Geometry check sheet. Reference: drawing and pictorial views, mm from the part's lowest x, y, z. Give positions to 0.01 mm unless a question says otherwise; leave off trailing zeros. Write each loop counter-clockwise with the first axis right and the second up, starting at its lowest first coordinate (ties: lowest second). Pieces come first, ordered by that corner, then holes. Notation, with made-up numbers: M 76.5,58.5 L 104.5,58.5 A17 cw 104.5,63.5 Z; hole C 84,12 d5. An arc over 180 degrees is marked long. One line per item, written item: value. Start each with the question number.
1. Cross-section at B-B on x = 6.25. Record the cut outline in (y, z), then the cut area to 3 significant figures.
2. Cross-section at A-A on y = 1.7. Record the cut outline in (x, z), then the cut area to 3 significant figures.
3. Scan lines: line 1 (Z direction, x = 6, y = 3.2); line 2 (Z direction, x = 4.5, y = 1.1); line 3 (Y direction, x = 5, z = 7). Record each from-to range of solid material in increasing order.
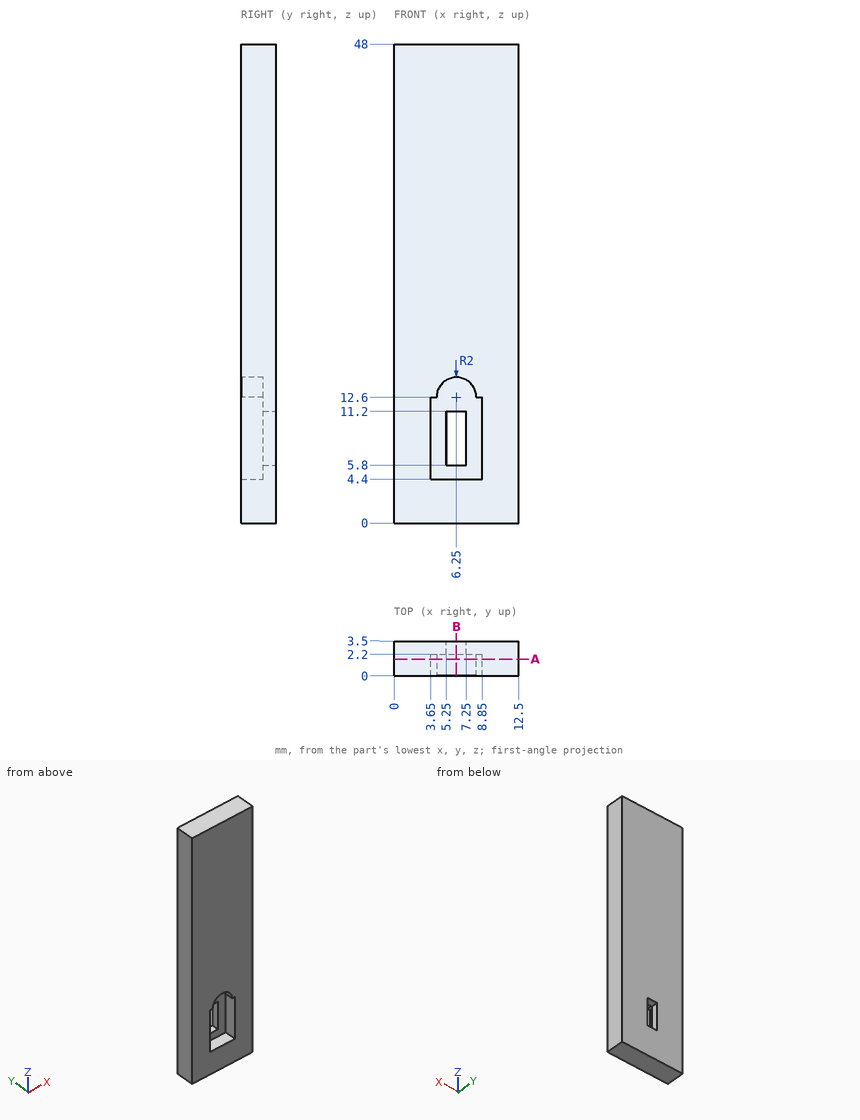
Report:
1. outline: M 0,0 L 3.5,0 L 3.5,5.8 L 2.2,5.8 L 2.2,4.4 L 0,4.4 Z; M 0,14.6 L 2.2,14.6 L 2.2,11.2 L 3.5,11.2 L 3.5,48 L 0,48 Z
1. area: 139 mm^2
2. outline: M 0,0 L 12.5,0 L 12.5,48 L 0,48 Z; hole M 3.65,4.4 L 8.85,4.4 L 8.85,12.6 L 8.25,12.6 A2 ccw 4.25,12.6 L 3.65,12.6 Z
2. area: 551 mm^2
3. line 1: z = 0 to 5.8, 11.2 to 48
3. line 2: z = 0 to 4.4, 13.57 to 48
3. line 3: y = 2.2 to 3.5
